Design review of the part built by this model. Coordinates are the model's own, in mm. Give positions to 0.01 mm unless a question says otherwise; leave off trailing zeros. Write each loop counter-clockwise with the first axis right and the second up, starting at its lowest first coordinate (ties: lowest second). Pieces come first, ordered by that corner, then holes. Notation, with made-up numbers: (46.5, 21.25) -> (59.5, 21.25) arc R24 cw to (59.5, 59.25) -> close; hole circle Ø2 at (-30.5, 9). An arc over 180 degrees is marked (long way). Answer as a JSON object with one key per item and string values.
```python
from build123d import *

# Parameters (mm, degrees)
SKETCH1_W                     = 45
SKETCH1_H                     = 43
BOSS_EXTRUDE1_DEPTH           = 153
SKETCH2_R                     = 2.5
BOSS_EXTRUDE4_DEPTH           = 7
SKETCH3_R                     = 2.5
BOSS_EXTRUDE5_DEPTH           = 7
BOSS_EXTRUDE5_DRAFT           = 15
BOSS_EXTRUDE5_PROFILE_2_DEPTH = 7
BOSS_EXTRUDE5_PROFILE_2_DRAFT = 15


with BuildPart() as part:
    # Sketch1 → Boss-Extrude1 (new body)
    with BuildSketch(Plane(origin=(0, 0, 0), x_dir=(1, 0, 0), z_dir=(0, 1, 0))):
        Rectangle(SKETCH1_W, SKETCH1_H)
    extrude(amount=BOSS_EXTRUDE1_DEPTH)

    # Sketch2 → Boss-Extrude4 (add)
    with BuildSketch(Plane(origin=(0, 153, 0), x_dir=(1, 0, 0), z_dir=(0, 1, 0))):
        with Locations(Location((22.5, -2.55, 0), (0, 0, 270))):
            Circle(SKETCH2_R)
        with Locations(Location((22.5, 2.55, 0), (0, 0, 270))):
            Circle(SKETCH2_R)
    extrude(amount=BOSS_EXTRUDE4_DEPTH)


with BuildPart() as boss_extrude5_tool:
    # Sketch3 → Boss-Extrude5 (with draft: the straight prism first)
    with BuildSketch(Plane.XZ.offset(-153)):
        with Locations(Location((22.5, 2.55, 0), (0, 0, 90))):
            Circle(SKETCH3_R)
    extrude(amount=BOSS_EXTRUDE5_DEPTH)
    # Boss-Extrude5: the draft: its side faces are tilted about the plane it starts from
    boss_extrude5_sides = [boss_extrude5_tool.faces().sort_by_distance(p)[0] for p in [
        (22.5, 149.5, 0.05),
    ]]
    draft(boss_extrude5_sides, Plane.XZ.offset(-153), BOSS_EXTRUDE5_DRAFT)


with BuildPart() as part_1:
    add(part.part)

    # Boss-Extrude5: add boss_extrude5_tool
    add(boss_extrude5_tool.part)


with BuildPart() as boss_extrude5_profile_2_tool:
    # Sketch3 → Boss-Extrude5 profile 2 (with draft: the straight prism first)
    with BuildSketch(Plane.XZ.offset(-153)):
        with Locations(Location((22.5, -2.55, 0), (0, 0, 90))):
            Circle(SKETCH3_R)
    extrude(amount=BOSS_EXTRUDE5_PROFILE_2_DEPTH)
    # Boss-Extrude5 profile 2: the draft: its side faces are tilted about the plane it starts from
    boss_extrude5_profile_2_sides = [boss_extrude5_profile_2_tool.faces().sort_by_distance(p)[0] for p in [
        (22.5, 149.5, -5.05),
    ]]
    draft(boss_extrude5_profile_2_sides, Plane.XZ.offset(-153), BOSS_EXTRUDE5_PROFILE_2_DRAFT)


with BuildPart() as part_2:
    add(part_1.part)

    # Boss-Extrude5 profile 2: add boss_extrude5_profile_2_tool
    add(boss_extrude5_profile_2_tool.part)


solid = part_2.part
```
(1) Clearance check with flat-ended pins moving along their axes: pin 1 (0.5 mm diameter, centred on x = 23, z = -2.5, fed in from -Y); pin 2 (5 mm diameter, centred on x = -2.5, z = 14.5, fed in from -Y); pin 3 (21.5 mm diameter, centred on x = -0.5, z = 1, fed in from +Y); pin 4 (12 mm diameter, centred on y = 95, z = -17, fed in from +X). State where each tip first meets the part, or that it passes through.
Here are the results:
{"pin 1": "stops at y = 146", "pin 2": "stops at y = 0", "pin 3": "stops at y = 153", "pin 4": "stops at x = 22.5"}
(2) We need section A-A, the plane z = 16.5. State the section outline as (x, y) points, then the cut area to 4 significant figures.
Here are the results:
{"outline": "(-22.5, 0) -> (22.5, 0) -> (22.5, 153) -> (-22.5, 153) -> close", "area": "6,885 mm²"}
(3) The part is to be moulded in two halves that separate along Z. For faces 1 (the flat face through (0, 75, 21.5)), 2 (the flat face through (23, 160, 3)), 3 (the conical face through (24.075, 149.549, -2.585)), say which applies: +Z half, -Z half, draft (parallel to the pull), parting line (faces both ways), or undercut.
Here are the results:
{"face 1": "+Z half", "face 2": "draft", "face 3": "undercut"}
(4) For line 1 along X through (y, z) = (129, -6); line 2 along Y through (x, z) = (-13.5, -19), list the stretches that pass through material, from the lowest coordinate up.
Here are the results:
{"line 1": "x = -22.5 to 22.5", "line 2": "y = 0 to 153"}
(5) We need section B-B, the plane y = 35.5. State the section outline as (x, z) points.
Here are the results:
{"outline": "(-22.5, -21.5) -> (22.5, -21.5) -> (22.5, 21.5) -> (-22.5, 21.5) -> close"}
